Work out the finished part from the listing and answer in its coordinate system (mm). A direction names the side the tool comes from. Coordinates: 2 decimals unless noted, no trailing zeros. Order: outer loops, then holes, each group sorted by start corner. A loop starts at its lowest first (then second) coordinate and runs counter-clockwise, first axis right, second up.
1. A tool of negligible diameter and unlimited length cuts with its end or side. For faces 4 (the flat face through (-1, 20, 6)), 5 (the flat face through (1, 20, 6)), 6 (the flat face through (25, -1, 0)), 7 (the flat face through (-25, -1, 0)), 8 (the cylindrical face through (-0.464, -24.724, 17.039)), from which of +Z, -Z, +X, -X, +Y, -Y can it reach the whole face along a straight path? Write none if from no direction.
2. The part is cut by section A-A, the plane x = 0. Give the vertices of the cut face in (y, z).
3. The part is cut by section B-B, the plane z = 6. Give the vertices of the cut face in (x, y).
4. Find the intervals of material crossed by probe 1 along Z at (x, y) = (-8, -4.5); probe 2 along Y at (x, z) = (0, 7.5), in increasing order.
5. Flat-ended cylindrical pins translate along their axes: pin 1 Ø8 at (x, y) = (-2.5, -15.5) entering from +Z; pin 2 Ø1 at (y, z) = (19, 6.5) entering from -X; pin 3 Ø12 at (y, z) = (23, 18) entering from -X; pin 4 Ø1 at (y, z) = (20, 5.5) entering from +X. Find the tip coordinate at first contact, or state that the pin passes through.
6. The part is cut by section D-D, the plane x = 12.5. Give the vertices of the cut face in (y, z).
7. Determine the mould class of faces 1 (the cylindrical face through (0.014, 20.104, 7.912)), 2 (the flat face through (0, 36.139, 0)), 3 (the flat face through (0, -23, 29.714)) for opening direction Y: +Y half, -Y half, draft (parallel to the pull), parting line (faces both ways), or undercut.
8. The part is cut by section C-C, the plane y = -5.5. Give the vertices of the cut face in (x, z).
```python
from build123d import *

# Parameters (mm, degrees)
F0_W     = 72.277866
F0_H     = 9.427548
F1_DEPTH = 25
F2_R     = 2.140903
F3_DEPTH = 25
F4_R     = 3.199453
F5_DEPTH = 1


with BuildPart() as f1:
    # F0 (on Right) → F1 (new body, symmetric)
    with BuildSketch(Plane.YZ):
        Rectangle(F0_W, F0_H)
    extrude(amount=F1_DEPTH, both=True)

    # F2 (on face) → F3 (join)
    with BuildSketch(Plane.XY.offset(4.713774)):
        with Locations((0, -22.634452)):
            Circle(F2_R)
    extrude(amount=F3_DEPTH)

    # F4 (on Right) → F5 (join, symmetric)
    with BuildSketch(Plane.YZ):
        with Locations((20.03381, 4.713774)):
            Circle(F4_R)
    extrude(amount=F5_DEPTH, both=True)


solid = f1.part
```
Geometry says:
1. face 4: +Z, -X, +Y
1. face 5: +Z, +X, +Y
1. face 6: +Z, -Z, +X, +Y, -Y
1. face 7: +Z, -Z, -X, +Y, -Y
1. face 8: +Z
2. outline: (-36.14, -4.71) - (36.14, -4.71) - (36.14, 4.71) - (23.23, 4.71) arc R3.2 ccw to (16.83, 4.71) - (-20.49, 4.71) - (-20.49, 29.71) - (-24.78, 29.71) - (-24.78, 4.71) - (-36.14, 4.71) - close
3. outline: circle Ø4.28 at (0, -22.63); (-1, 17.1) - (1, 17.1) - (1, 22.96) - (-1, 22.96) - close
4. probe 1: z = -4.71 to 4.71
4. probe 2: y = -24.78 to -20.49, 18.46 to 21.61
5. pin 1: stops at z = 4.71
5. pin 2: stops at x = -1
5. pin 3: passes through
5. pin 4: stops at x = 1
6. outline: (-36.14, -4.71) - (36.14, -4.71) - (36.14, 4.71) - (-36.14, 4.71) - close
7. face 1: undercut
7. face 2: +Y half
7. face 3: draft
8. outline: (-25, -4.71) - (25, -4.71) - (25, 4.71) - (-25, 4.71) - close
